The model under review builds one solid part; all positions refer to its coordinate system, in mm. A direction names the side the tool comes from. Give positions to 0.01 mm unless a question says otherwise; leave off trailing zeros. Write each loop counter-clockwise with the first axis right and the second up, starting at its lowest first coordinate (ties: lowest second). Pieces come first, ordered by that corner, then holes. Notation, with made-up numbers: (-26, 64) - (-8, 64) arc R24 ccw to (-8, 74) - close; hole circle Ø10 at (46.25, 27.5). An arc over 180 degrees is marked (long way). Write item = value, one per line.
Autodesk Inventor part; units mm, degrees
ref_plane "YZ Plane" through (0, 0, 0) normal (1, 0, 0) x (0, 1, 0)
ref_plane "XZ Plane" through (0, 0, 0) normal (0, 1, 0) x (-1, 0, 0)
ref_plane "XY Plane" through (0, 0, 0) normal (0, 0, 1) x (1, 0, 0)
sketch "Sketch1" plane through (0, 0, 0) normal (0, 0, 1) x (1, 0, 0)
  circle A0 centre (0, 0) radius 100
  circle A1 centre (0, 0) radius 80
  line L0 (-26.6667, -55.5556) -> (-26.6667, 55.5556)
  line L1 (-26.6667, 55.5556) -> (10, 55.5556)
  arc A2 (10, -11.1111) -> (10, 55.5556) centre (10, 22.2222) ccw
  line L2 (10, -11.1111) -> (-6.6667, -11.1111)
  line L3 (-6.6667, -11.1111) -> (-6.6667, -55.5556)
  line L4 (-6.6667, -55.5556) -> (-26.6667, -55.5556)
  line L5 (-6.6667, 35.5556) -> (10, 35.5556)
  arc A3 (10, 8.8889) -> (10, 35.5556) centre (10, 22.2222) ccw
  line L6 (10, 8.8889) -> (-6.6667, 8.8889)
  line L7 (-6.6667, 8.8889) -> (-6.6667, 35.5556)
  line L8 (-34.0741, 11.8519) -> (50.7407, 11.8519)
  line L9 (50.7407, 11.8519) -> (50.7407, 19.2593)
  line L10 (50.7407, 19.2593) -> (-34.0741, 19.2593)
  line L11 (-34.0741, 19.2593) -> (-34.0741, 11.8519)
  line L12 (-34.0741, 25.1852) -> (50.7407, 25.1852)
  line L13 (50.7407, 25.1852) -> (50.7407, 32.5926)
  line L14 (50.7407, 32.5926) -> (-34.0741, 32.5926)
  line L15 (-34.0741, 32.5926) -> (-34.0741, 25.1852)
  line L16 (1.6667, 8.8889) -> (1.6667, 32.5926) construction
  line L17 (1.6667, 35.5556) -> (1.6667, 11.8519) construction
  line L18 (0, 80) -> (0, 55.5556) construction
  line L19 (0, -80) -> (0, -11.1111) construction
  line L20 (-26.6667, 0) -> (0, 0) construction
  line L21 (50.7407, 25.1852) -> (50.7407, 19.2593) construction
  line L22 (50.7407, 22.2222) -> (10, 22.2222) construction
  line L23 (43.3333, 22.2222) -> (50.7407, 22.2222) construction
  point P0 (0, -45.5556)
  dimension "d0" = 20
  dimension "d1" = 200
  dimension "d2" = 20
  dimension "d3" = 20
  dimension "d4" = 7.4074
  dimension "d5" = 111.1111
  dimension "d6" = 2.963
  dimension "d7" = 7.4074
  dimension "d12" = 7.4074
  dimension "d50" = 44.4444
  dimension "d52" = 10
  dimension "d53" = 30
extrude "Extrusion1" add sketch "Sketch1" along normal blind 10 contours A0 | L0 L8 L7 L6 A3 A2 L2 L3 L4 | L0 L10 L7 L8 | L0 L12 L7 L10 | L0 L14 L7 L12 | A3 L10 A2 L8 | L0 L1 A2 L14 A3 L5 L7 | A3 L12 A2 L10 | A3 L14 A2 L12
sketch "Sketch2" plane through (0, 0, 10) normal (0, 0, 1) x (1, 0, 0)
  line L0 (-34.0741, 25.1852) -> (50.7407, 25.1852)
  line L1 (50.7407, 32.5926) -> (-34.0741, 32.5926)
  line L2 (50.7407, 25.1852) -> (50.7407, 32.5926)
  line L3 (-34.0741, 32.5926) -> (-34.0741, 25.1852)
  line L4 (50.7407, 19.2593) -> (-34.0741, 19.2593)
  line L5 (-34.0741, 19.2593) -> (-34.0741, 11.8519)
  line L6 (-34.0741, 11.8519) -> (50.7407, 11.8519)
  line L7 (50.7407, 11.8519) -> (50.7407, 19.2593)
  point P0 (0, 0)
extrude "Extrusion2" add sketch "Sketch2" against normal blind 4
sketch "Sketch3" plane through (0, 0, 0) normal (0, 0, -1) x (-1, 0, 0)
  circle A0 centre (0, 0) radius 100
extrude "Extrusion3" add sketch "Sketch3" along normal blind 5
fillet "Fillet2" radius 2 2 edges at (-6.6667, 8.8889, 5) (-6.6667, 35.5556, 5)
fillet "Fillet3" radius 2 1 edges at (-6.6667, -11.1111, 5)
chamfer "Chamfer1" distance 0.5 angle 45 3 edges at (-26.6667, 55.5556, 5) (-26.6667, -55.5556, 5) (-6.6667, -55.5556, 5)
sketch "Sketch6" plane through (0, 0, 10) normal (0, 0, 1) x (1, 0, 0)
  line L0 (50.7407, 32.5926) -> (-34.0741, 32.5926)
  line L1 (-34.0741, 32.5926) -> (-34.0741, 25.1852)
  line L2 (-34.0741, 25.1852) -> (50.7407, 25.1852)
  line L3 (50.7407, 25.1852) -> (50.7407, 32.5926)
  line L4 (-34.0741, 19.2593) -> (50.7407, 19.2593)
  line L5 (50.7407, 19.2593) -> (50.7407, 11.8519)
  line L6 (50.7407, 11.8519) -> (-34.0741, 11.8519)
  line L7 (-34.0741, 11.8519) -> (-34.0741, 19.2593)
  point P0 (0, 0)
extrude "Extrusion5" add sketch "Sketch6" along normal blind 4
equation "\"d0\" = 0.1 * d1"
equation "\"d2\" = d0"
equation "\"d3\" = d2"
equation "\"d4\" = 0.0666667 * d5"
equation "\"d5\" = 0.555556 * d1"
equation "\"d6\" = 0.4 * d4"
equation "\"d7\" = d4"
equation "\"d12\" = d4"
equation "\"d50\" = 0.4 * d5"
equation "\"d53\" = 3 * d52"
properties part number "PennyKoin-3D-Inventor"
1. Take a section at C-C on x = -20. Give the boundary of the cut face in (y, z).
Findings below:
outline = (-97.98, -5) - (97.98, -5) - (97.98, 10) - (77.46, 10) - (77.46, 0) - (55.56, 0) - (55.56, 10) - (32.59, 10) - (32.59, 14) - (25.19, 14) - (25.19, 10) - (19.26, 10) - (19.26, 14) - (11.85, 14) - (11.85, 10) - (-55.56, 10) - (-55.56, 0) - (-77.46, 0) - (-77.46, 10) - (-97.98, 10) - close
2. For line 1 (Y direction, x = 0, z = 2); line 2 (Y direction, x = 3.5, z = 9.75); line 3 (Y direction, x = 0, z = 8.25), list the stretches that pass through material, from the lowest coordinate up. Write a range as from..to.
Findings below:
line_1 = -100..-80, -11.11..8.89, 35.56..55.56, 80..100
line_2 = -99.94..-79.92, -11.11..8.89, 11.85..19.26, 25.19..32.59, 35.56..55.56, 79.92..99.94
line_3 = -100..-80, -11.11..8.89, 11.85..19.26, 25.19..32.59, 35.56..55.56, 80..100
3. Insertion check: P1, Ø2, axis at y = 15, z = 8, coming from the +X side; P2, Ø8, axis at x = -19.5, z = 3.5, coming from the -Y side; P3, Ø5, axis at x = -4.5, z = 3, coming from the +Y side. Each pin has a flat end and moves straight along its axis. Give the tip position at first contact, or say it passes through.
Findings below:
P1 = 99.02
P2 = -98.79
P3 = 99.98
4. Machinability: for faces 1 (the flat face through (-8, -14, 10)), 2 (the flat face through (-6.667, -34, 5)), 3 (the flat face through (-30, 16, 6)), 4 (the flat face through (1, 1, -5)), which of the approach directions +Z, -Z, +X, -X, +Y, -Y give a long, thin tool a straight path to every point of the face, cutting with its end or side? Answer none if there is none.
Findings below:
face_1 = +Z, +X, -X, -Y
face_2 = +Z
face_3 = none
face_4 = -Z, +X, -X, +Y, -Y
5. Take a section at D-D on z = -2.5. Give the boundary of the cut face in (x, y).
Findings below:
outline = circle Ø200 at (0, 0)
6. Draft analysis for pull direction Z (two halves, no side actions). For faces 5 (the flat face through (8, 16, 14)), 6 (the flat face through (46, 29, 6)), 7 (the flat face through (3, 35.556, 5)), 8 (the flat face through (8, 16, 6)), state which applies: +Z half, -Z half, draft (parallel to the pull), parting line (faces both ways), or undercut.
Findings below:
face_5 = +Z half
face_6 = undercut
face_7 = draft
face_8 = undercut
7. Take a section at B-B on y = 0. Give the boundary of the cut face in (x, z), and give its area (3 significant figures).
Findings below:
outline = (-100, -5) - (100, -5) - (100, 10) - (80, 10) - (80, 0) - (34.85, 0) - (34.85, 10) - (-26.67, 10) - (-26.67, 0) - (-80, 0) - (-80, 10) - (-100, 10) - close
area = 2,020 mm²
8. Take a section at A-A on x = 0. Give the boundary of the cut face in (y, z).
Findings below:
outline = (-100, -5) - (100, -5) - (100, 10) - (80, 10) - (80, 0) - (55.56, 0) - (55.56, 10) - (35.56, 10) - (35.56, 0) - (8.89, 0) - (8.89, 10) - (-11.11, 10) - (-11.11, 0) - (-80, 0) - (-80, 10) - (-100, 10) - close; (11.85, 6) - (19.26, 6) - (19.26, 14) - (11.85, 14) - close; (25.19, 6) - (32.59, 6) - (32.59, 14) - (25.19, 14) - close
